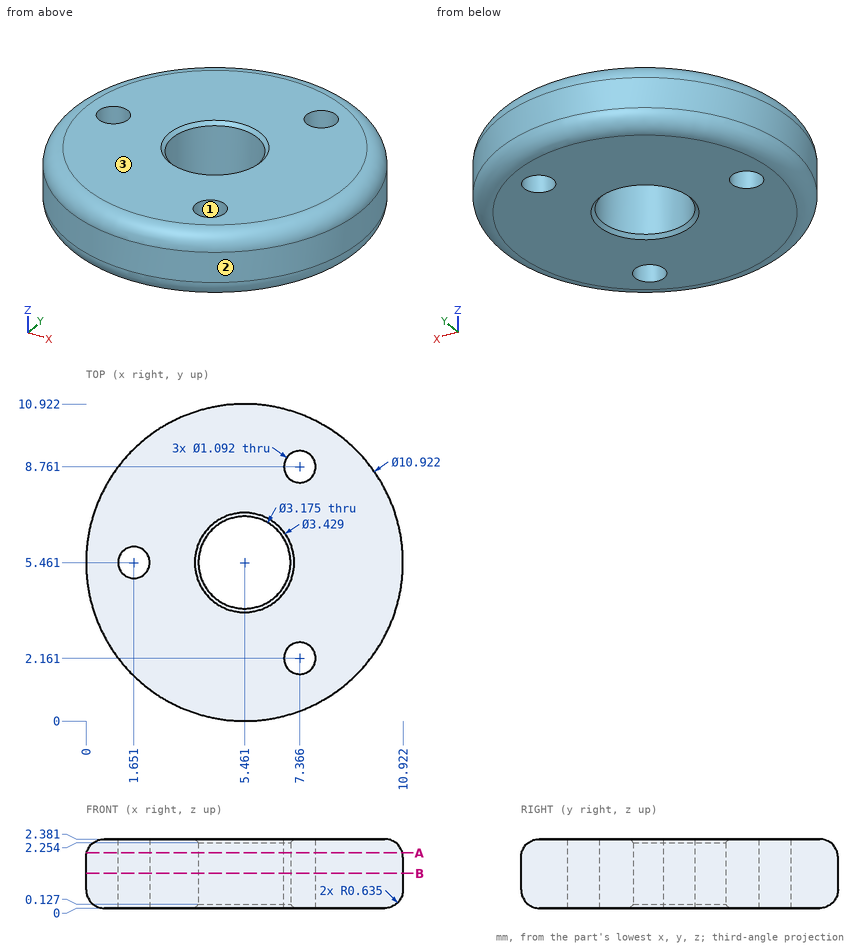
Here's the drawing with two shaded views (mm, measured from the low corner). I have some questions. Give positions to 0.01 mm unless a question says otherwise; leave off trailing zeros. Write each loop counter-clockwise with the first axis right and the second up, starting at its lowest first coordinate (ties: lowest second). Pieces come first, ordered by that corner, then holes. Notation, with made-up numbers: (-17, 63) -> (42, 63) arc R8 cw to (42, 72) -> close; hole circle Ø6 at (6, 41.25). An arc over 180 degrees is marked (long way). Answer as a JSON object with one key per item and string values. Group by question number.
Item 1: Please list where these lines run through material, in increasing order: line 1 (X direction, y = 5.25, z = 1.65) (1 decimal); line 2 (X direction, y = 4.5, z = 2.15) (1 decimal); line 3 (X direction, y = 8.75, z = 0.45) (1 decimal). Write a range as [from, to].
Item 2: Suppose I cut it at A-A (z = 1.9). Please give me the cut outline in (x, y) (1 decimal).
Item 3: We'd pull the mould along Y, two halves only. Please class the marked faces 1, 2 and 3: +Y half, -Y half, draft (parallel to the pull), parting line (faces both ways), or undercut.
Item 4: I'm going to push a flat-ended pin straight in: P1, Ø1, axis at x = 7.37, y = 2.16, coming from the +Z side. Where does the tip first touch, or does it pass through?
Findings:
{
 "1": {"line 1": "x = [0, 1.1], [2.2, 3.9], [7, 10.9]", "line 2": "x = [0.2, 4.2], [6.7, 10.7]", "line 3": "x = [1.1, 6.8], [7.9, 9.8]"},
 "2": {"outline": "circle Ø10.9 at (5.5, 5.5); hole circle Ø1.1 at (1.7, 5.5); hole circle Ø3.2 at (5.5, 5.5); hole circle Ø1.1 at (7.4, 2.2); hole circle Ø1.1 at (7.4, 8.8)"},
 "3": {"face 1": "undercut", "face 2": "parting line", "face 3": "draft"},
 "4": {"P1": "passes through"}
}
